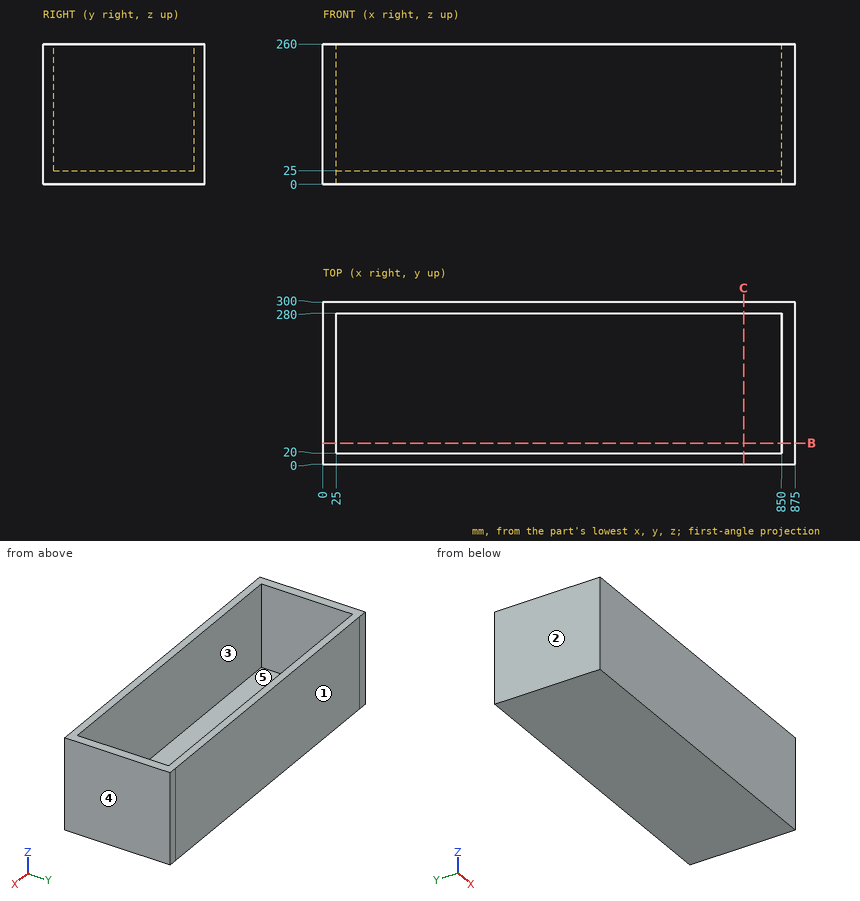
Geometry check sheet. Reference: drawing and pictorial views, mm from the part's lowest x, y, z. A direction names the side the tool comes from. Give positions to 0.01 mm unless a question says otherwise; leave off trailing zeros. Order: outer loops, then holes, each group sorted by start corner. A loop starts at its lowest first (then second) coordinate and runs counter-clockwise, first axis right, second up. Notation, with made-up numbers: (28.5, 83) - (36.5, 83) arc R17 cw to (36.5, 110) - close; hole circle Ø6 at (55, 55.5). An arc over 180 degrees is marked (long way). Answer as CSV lines item,"result".
1. Mould release check, pull along Y, two halves, no side actions. Record for the marked faces 1, 2 and 3: released by +Y, released by -Y, zero draft, split by the parting line, or undercut.
Result sheet:
face 1,"released by +Y"
face 2,"zero draft"
face 3,"undercut"
2. Section check B-B (y = 39). Record the boundary of the cut face in (x, z), then the cut area to 3 significant figures.
Result sheet:
outline,"(0, 0) - (875, 0) - (875, 260) - (850, 260) - (850, 25) - (25, 25) - (25, 260) - (0, 260) - close"
area,"33,600 mm²"
3. Go/stop test with flat-tipped pins: P1, Ø1, axis at x = 205, y = 129.5, coming from the +Z side; P2, Ø5, axis at y = 262, z = 164, coming from the -X side. Record where each tip stops, or that it passes through.
Result sheet:
P1,"z = 25"
P2,"x = 0"
4. Section check C-C (x = 780). Record the boundary of the cut face in (y, z), then the cut area to 3 significant figures.
Result sheet:
outline,"(0, 0) - (300, 0) - (300, 260) - (280, 260) - (280, 25) - (20, 25) - (20, 260) - (0, 260) - close"
area,"16,900 mm²"
5. Scan lines: probe 1 along X at (y, z) = (46.5, 109); probe 2 along Y at (x, z) = (51.5, 35.5); probe 3 along Z at (x, y) = (625.5, 212.5). Record each from-to range of solid material in increasing order. Write a range as from..to.
Result sheet:
probe 1,"0..25, 850..875"
probe 2,"0..20, 280..300"
probe 3,"0..25"
6. Tool access check on the marked faces 4 and 5. Record the directions out of +Z, -Z, +X, -X, +Y, -Y that give a thin tool (end or side, any length) a straight path to the whole face; none if there is none.
Result sheet:
face 4,"+Z, -Z, +X, +Y, -Y"
face 5,"+Z"
